Part model, mm, in its own coordinate system. Face numbers are marked on the shaded views. A direction names the side the tool comes from. Coordinates: 2 decimals unless noted, no trailing zeros. Order: outer loops, then holes, each group sorted by start corner. A loop starts at its lowest first (then second) coordinate and runs counter-clockwise, first axis right, second up.
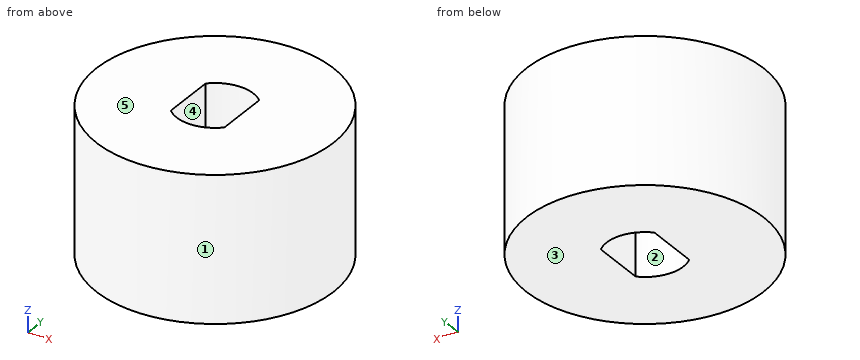
Autodesk Inventor part; units mm, degrees
ref_plane "YZ Plane" through (0, 0, 0) normal (1, 0, 0) x (0, 1, 0)
ref_plane "XZ Plane" through (0, 0, 0) normal (0, 1, 0) x (-1, 0, 0)
ref_plane "XY Plane" through (0, 0, 0) normal (0, 0, 1) x (1, 0, 0)
sketch "Sketch1" plane through (0, 0, 0) normal (0, 0, 1) x (1, 0, 0)
  line L0 (0.2752, -3.536) -> (0.7321, -4.3005)
  arc A0 (0.5159, -4.5981) -> (0.7321, -4.3005) centre (0.5604, -4.4031) ccw
  line L1 (0.5159, -4.5981) -> (-0.3524, -4.3999)
  arc A1 (-0.3524, -4.3999) -> (-0.5862, -4.6595) centre (-0.3969, -4.5949) ccw
  line L2 (-0.5862, -4.6595) -> (-0.2983, -5.5023)
  arc A2 (-0.5716, -5.7484) -> (-0.2983, -5.5023) centre (-0.4875, -5.5669) ccw
  line L3 (-0.5716, -5.7484) -> (-1.3796, -5.374)
  arc A3 (-1.3796, -5.374) -> (-1.6623, -5.5793) centre (-1.4637, -5.5554) ccw
  line L4 (-1.6623, -5.5793) -> (-1.5559, -6.4635)
  arc A4 (-1.8745, -6.6475) -> (-1.5559, -6.4635) centre (-1.7545, -6.4874) ccw
  line L5 (-1.8745, -6.6475) -> (-2.587, -6.1132)
  arc A5 (-2.587, -6.1132) -> (-2.9062, -6.2553) centre (-2.707, -6.2732) ccw
  line L6 (-2.9062, -6.2553) -> (-2.9859, -7.1423)
  arc A6 (-3.3358, -7.256) -> (-2.9859, -7.1423) centre (-3.1851, -7.1244) ccw
  line L7 (-3.3358, -7.256) -> (-3.9217, -6.5853)
  arc A7 (-3.9217, -6.5853) -> (-4.2634, -6.6579) centre (-4.0723, -6.7169) ccw
  line L8 (-4.2634, -6.6579) -> (-4.5259, -7.5089)
  arc A8 (-4.8917, -7.5474) -> (-4.5259, -7.5089) centre (-4.717, -7.45) ccw
  line L9 (-4.8917, -7.5474) -> (-5.3253, -6.7695)
  arc A9 (-5.3253, -6.7695) -> (-5.6747, -6.7695) centre (-5.5, -6.8669) ccw
  line L10 (-5.6747, -6.7695) -> (-6.1083, -7.5474)
  arc A10 (-6.4741, -7.5089) -> (-6.1083, -7.5474) centre (-6.283, -7.45) ccw
  line L11 (-6.4741, -7.5089) -> (-6.7366, -6.6579)
  arc A11 (-6.7366, -6.6579) -> (-7.0783, -6.5853) centre (-6.9277, -6.7169) ccw
  line L12 (-7.0783, -6.5853) -> (-7.6642, -7.256)
  arc A12 (-8.0141, -7.1423) -> (-7.6642, -7.256) centre (-7.8149, -7.1244) ccw
  line L13 (-8.0141, -7.1423) -> (-8.0938, -6.2553)
  arc A13 (-8.0938, -6.2553) -> (-8.413, -6.1132) centre (-8.293, -6.2732) ccw
  line L14 (-8.413, -6.1132) -> (-9.1255, -6.6475)
  arc A14 (-9.4441, -6.4635) -> (-9.1255, -6.6475) centre (-9.2455, -6.4874) ccw
  line L15 (-9.4441, -6.4635) -> (-9.3377, -5.5793)
  arc A15 (-9.3377, -5.5793) -> (-9.6204, -5.374) centre (-9.5363, -5.5554) ccw
  line L16 (-9.6204, -5.374) -> (-10.4284, -5.7484)
  arc A16 (-10.7017, -5.5023) -> (-10.4284, -5.7484) centre (-10.5125, -5.5669) ccw
  line L17 (-10.7017, -5.5023) -> (-10.4138, -4.6595)
  arc A17 (-10.4138, -4.6595) -> (-10.6476, -4.3999) centre (-10.6031, -4.5949) ccw
  line L18 (-10.6476, -4.3999) -> (-11.5159, -4.5981)
  arc A18 (-11.7321, -4.3005) -> (-11.5159, -4.5981) centre (-11.5604, -4.4031) ccw
  line L19 (-11.7321, -4.3005) -> (-11.2752, -3.536)
  arc A19 (-11.2752, -3.536) -> (-11.4499, -3.2335) centre (-11.4469, -3.4335) ccw
  line L20 (-11.4499, -3.2335) -> (-12.3404, -3.2469)
  arc A20 (-12.49, -2.9108) -> (-12.3404, -3.2469) centre (-12.3434, -3.0469) ccw
  line L21 (-12.49, -2.9108) -> (-11.8842, -2.258)
  arc A21 (-11.8842, -2.258) -> (-11.9922, -1.9258) centre (-12.0308, -2.122) ccw
  line L22 (-11.9922, -1.9258) -> (-12.866, -1.7537)
  arc A22 (-12.9425, -1.3939) -> (-12.866, -1.7537) centre (-12.8273, -1.5575) ccw
  line L23 (-12.9425, -1.3939) -> (-12.2142, -0.8813)
  arc A23 (-12.2142, -0.8813) -> (-12.2507, -0.5339) centre (-12.3293, -0.7178) ccw
  line L24 (-12.2507, -0.5339) -> (-13.0696, -0.1839)
  arc A24 (-13.0696, 0.1839) -> (-13.0696, -0.1839) centre (-12.991, 0) ccw
  line L25 (-13.0696, 0.1839) -> (-12.2507, 0.5339)
  arc A25 (-12.2507, 0.5339) -> (-12.2142, 0.8813) centre (-12.3293, 0.7178) ccw
  line L26 (-12.2142, 0.8813) -> (-12.9425, 1.3939)
  arc A26 (-12.866, 1.7537) -> (-12.9425, 1.3939) centre (-12.8273, 1.5575) ccw
  line L27 (-12.866, 1.7537) -> (-11.9922, 1.9258)
  arc A27 (-11.9922, 1.9258) -> (-11.8842, 2.258) centre (-12.0308, 2.122) ccw
  line L28 (-11.8842, 2.258) -> (-12.49, 2.9108)
  arc A28 (-12.3404, 3.2469) -> (-12.49, 2.9108) centre (-12.3434, 3.0469) ccw
  line L29 (-12.3404, 3.2469) -> (-11.4499, 3.2335)
  arc A29 (-11.4499, 3.2335) -> (-11.2752, 3.536) centre (-11.4469, 3.4335) ccw
  line L30 (-11.2752, 3.536) -> (-11.7321, 4.3005)
  arc A30 (-11.5159, 4.5981) -> (-11.7321, 4.3005) centre (-11.5604, 4.4031) ccw
  line L31 (-11.5159, 4.5981) -> (-10.6476, 4.3999)
  arc A31 (-10.6476, 4.3999) -> (-10.4138, 4.6595) centre (-10.6031, 4.5949) ccw
  line L32 (-10.4138, 4.6595) -> (-10.7017, 5.5023)
  arc A32 (-10.4284, 5.7484) -> (-10.7017, 5.5023) centre (-10.5125, 5.5669) ccw
  line L33 (-10.4284, 5.7484) -> (-9.6204, 5.374)
  arc A33 (-9.6204, 5.374) -> (-9.3377, 5.5793) centre (-9.5363, 5.5554) ccw
  line L34 (-9.3377, 5.5793) -> (-9.4441, 6.4635)
  arc A34 (-9.1255, 6.6475) -> (-9.4441, 6.4635) centre (-9.2455, 6.4874) ccw
  line L35 (-9.1255, 6.6475) -> (-8.413, 6.1132)
  arc A35 (-8.413, 6.1132) -> (-8.0938, 6.2553) centre (-8.293, 6.2732) ccw
  line L36 (-8.0938, 6.2553) -> (-8.0141, 7.1423)
  arc A36 (-7.6642, 7.256) -> (-8.0141, 7.1423) centre (-7.8149, 7.1244) ccw
  line L37 (-7.6642, 7.256) -> (-7.0783, 6.5853)
  arc A37 (-7.0783, 6.5853) -> (-6.7366, 6.6579) centre (-6.9277, 6.7169) ccw
  line L38 (-6.7366, 6.6579) -> (-6.4741, 7.5089)
  arc A38 (-6.1083, 7.5474) -> (-6.4741, 7.5089) centre (-6.283, 7.45) ccw
  line L39 (-6.1083, 7.5474) -> (-5.6747, 6.7695)
  arc A39 (-5.6747, 6.7695) -> (-5.3253, 6.7695) centre (-5.5, 6.8669) ccw
  line L40 (-5.3253, 6.7695) -> (-4.8917, 7.5474)
  arc A40 (-4.5259, 7.5089) -> (-4.8917, 7.5474) centre (-4.717, 7.45) ccw
  line L41 (-4.5259, 7.5089) -> (-4.2634, 6.6579)
  arc A41 (-4.2634, 6.6579) -> (-3.9217, 6.5853) centre (-4.0723, 6.7169) ccw
  line L42 (-3.9217, 6.5853) -> (-3.3358, 7.256)
  arc A42 (-2.9859, 7.1423) -> (-3.3358, 7.256) centre (-3.1851, 7.1244) ccw
  line L43 (-2.9859, 7.1423) -> (-2.9062, 6.2553)
  arc A43 (-2.9062, 6.2553) -> (-2.587, 6.1132) centre (-2.707, 6.2732) ccw
  line L44 (-2.587, 6.1132) -> (-1.8745, 6.6475)
  arc A44 (-1.5559, 6.4635) -> (-1.8745, 6.6475) centre (-1.7545, 6.4874) ccw
  line L45 (-1.5559, 6.4635) -> (-1.6623, 5.5793)
  arc A45 (-1.6623, 5.5793) -> (-1.3796, 5.374) centre (-1.4637, 5.5554) ccw
  line L46 (-1.3796, 5.374) -> (-0.5716, 5.7484)
  arc A46 (-0.2983, 5.5023) -> (-0.5716, 5.7484) centre (-0.4875, 5.5669) ccw
  line L47 (-0.2983, 5.5023) -> (-0.5862, 4.6595)
  arc A47 (-0.5862, 4.6595) -> (-0.3524, 4.3999) centre (-0.3969, 4.5949) ccw
  line L48 (-0.3524, 4.3999) -> (0.5159, 4.5981)
  arc A48 (0.7321, 4.3005) -> (0.5159, 4.5981) centre (0.5604, 4.4031) ccw
  line L49 (0.7321, 4.3005) -> (0.2752, 3.536)
  arc A49 (0.2752, 3.536) -> (0.4499, 3.2335) centre (0.4469, 3.4335) ccw
  line L50 (0.4499, 3.2335) -> (1.3404, 3.2469)
  arc A50 (1.49, 2.9108) -> (1.3404, 3.2469) centre (1.3434, 3.0469) ccw
  line L51 (1.49, 2.9108) -> (0.8842, 2.258)
  arc A51 (0.8842, 2.258) -> (0.9922, 1.9258) centre (1.0308, 2.122) ccw
  line L52 (0.9922, 1.9258) -> (1.866, 1.7537)
  arc A52 (1.9425, 1.3939) -> (1.866, 1.7537) centre (1.8273, 1.5575) ccw
  line L53 (1.9425, 1.3939) -> (1.2142, 0.8813)
  arc A53 (1.2142, 0.8813) -> (1.2507, 0.5339) centre (1.3293, 0.7178) ccw
  line L54 (1.2507, 0.5339) -> (2.0696, 0.1839)
  arc A54 (2.0696, -0.1839) -> (2.0696, 0.1839) centre (1.991, 0) ccw
  line L55 (2.0696, -0.1839) -> (1.2507, -0.5339)
  arc A55 (1.2507, -0.5339) -> (1.2142, -0.8813) centre (1.3293, -0.7178) ccw
  line L56 (1.2142, -0.8813) -> (1.9425, -1.3939)
  arc A56 (1.866, -1.7537) -> (1.9425, -1.3939) centre (1.8273, -1.5575) ccw
  line L57 (1.866, -1.7537) -> (0.9922, -1.9258)
  arc A57 (0.9922, -1.9258) -> (0.8842, -2.258) centre (1.0308, -2.122) ccw
  line L58 (0.8842, -2.258) -> (1.49, -2.9108)
  arc A58 (1.3404, -3.2469) -> (1.49, -2.9108) centre (1.3434, -3.0469) ccw
  line L59 (1.3404, -3.2469) -> (0.4499, -3.2335)
  arc A59 (0.4499, -3.2335) -> (0.2752, -3.536) centre (0.4469, -3.4335) ccw
  circle A60 centre (-5.5, 0) radius 5.5
  circle A61 centre (-5.5, 0) radius 5.5
  circle A62 centre (-5.5, 0) radius 3.15
  line L60 (-5.5, 0) -> (-4.6961, -7.6489)
  line L61 (-4.6961, -7.6489) -> (-4.5915, -8.6434)
  circle A63 centre (-5.5, 0) radius 8.691
  line L62 (-7.35, -1.8974) -> (-7.35, 1.8974)
  arc A64 (-7.35, -1.8974) -> (-3.65, -1.8974) centre (-5.5, 0) ccw
  line L63 (-3.65, 1.8974) -> (-3.65, -1.8974)
  arc A65 (-3.65, 1.8974) -> (-7.35, 1.8974) centre (-5.5, 0) ccw
  circle A66 centre (-5.5, 0) radius 1
  point P0 (0, 0)
  dimension "d0" = 1
extrude "Extrusion1" add sketch "Sketch1" along normal blind 10 contours A63 | A62 | A60 | L0 A0 L1 A1 L2 A2 L3 A3 L4 A4 L5 A5 L6 A6 L7 A7 L8 A8 L9 A9 L10 A10 L11 A11 L12 A12 L13 A13 L14 A14 L15 A15 L16 A16 L17 A17 L18 A18 L19 A19 L20 A20 L21 A21 L22 A22 L23 A23 L24 A24 L25 A25 L26 A26 L27 A27 L28 A28 L29 A29 L30 A30 L31 A31 L32 A32 L33 A33 L34 A34 L35 A35 L36 A36 L37 A37 L38 A38 L39 A39 L40 A40 L41 A41 L42 A42 L43 A43 L44 A44 L45 A45 L46 A46 L47 A47 L48 A48 L49 A49 L50 A50 L51 A51 L52 A52 L53 A53 L54 A54 L55 A55 L56 A56 L57 A57 L58 A58 L59 A59
sketch "Sketch2" plane through (-5.5, 0, 0) normal (0, 0, -1) x (-1, 0, 0)
  circle A0 centre (0, 0) radius 8.691
  arc A1 (-1.85, -1.8974) -> (1.85, -1.8974) centre (0, 0) ccw
  line L0 (-1.85, 1.8974) -> (-1.85, -1.8974)
  arc A2 (1.85, 1.8974) -> (-1.85, 1.8974) centre (0, 0) ccw
  line L1 (1.85, -1.8974) -> (1.85, 1.8974)
  circle A3 centre (0, 0) radius 8.691
  line L2 (0, -8.691) -> (0, -8.191)
  circle A4 centre (0, 0) radius 8.191
  point P0 (-5.5, 0)
  dimension "d3" = 0.5
extrude "Extrusion2" cut sketch "Sketch2" against normal through all contours A0
properties part number "kokoko"
(1) Probe line 1 (Y direction, x = -4.5, z = 5); line 2 (X direction, y = -2, z = 6.5); line 3 (Y direction, x = -5.25, z = 3). List the from-to ranges inside material, lowest first.
(2) Slice it at B-B, the plane x = -5.5. Give the cut face in (y, z).
(3) Slice it at A-A, the plane y = 0. Give the cut face in (x, z), then the cut area to 3 significant figures.
(4) Slice it at C-C, the plane z = 1. Give the cut face in (x, y).
(5) Drop a flat-ended pin along its axis: pin 1 (6 mm diameter, centred on x = -1, z = 6.5, fed in from +Y). Give the stop position or say it passes through.
(6) Tool access for the marked faces 4 and 5: list every direction of +Z, -Z, +X, -X, +Y, -Y with a clear straight run to the whole face (end or side of a thin tool).
(7) Pull direction X, two halves, no side cores. Call the marked faces 1, 2 and 3: +X half, -X half, draft (parallel to the pull), parting line (faces both ways), or undercut.
(8) Slice it at D-D, the plane y = -5.25. Give the cut face in (x, z), then the cut area to 3 significant figures.
Here are the results:
1. line 1: y = -8.13 to -2.45, 2.45 to 8.13
1. line 2: x = -13.44 to -7.24, -3.76 to 2.44
1. line 3: y = -8.19 to -2.64, 2.64 to 8.19
2. outline: (-8.19, 0) - (-2.65, 0) - (-2.65, 10) - (-8.19, 10) - close; (2.65, 0) - (8.19, 0) - (8.19, 10) - (2.65, 10) - close
3. outline: (-13.69, 0) - (-7.35, 0) - (-7.35, 10) - (-13.69, 10) - close; (-3.65, 0) - (2.69, 0) - (2.69, 10) - (-3.65, 10) - close
3. area: 127 mm2
4. outline: circle Ø16.38 at (-5.5, 0); hole (-7.35, -1.9) arc R2.65 ccw to (-3.65, -1.9) - (-3.65, 1.9) arc R2.65 ccw to (-7.35, 1.9) - close
5. pin 1: stops at y = 8.05
6. face 4: +Z, -Z
6. face 5: +Z, +X, -X, +Y, -Y
7. face 1: parting line
7. face 2: undercut
7. face 3: draft
8. outline: (-11.79, 0) - (0.79, 0) - (0.79, 10) - (-11.79, 10) - close
8. area: 126 mm2
